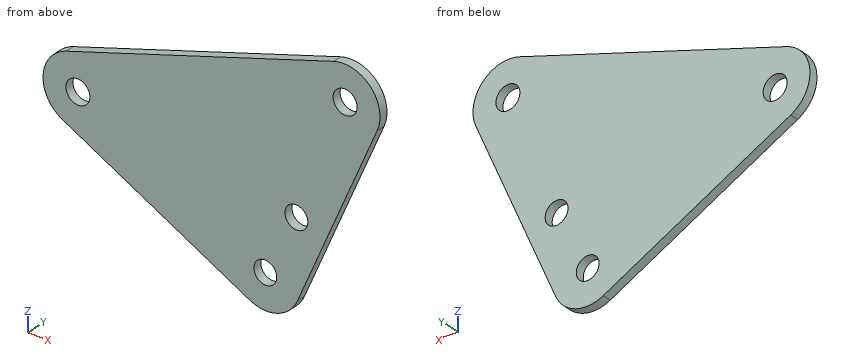
Autodesk Inventor part; units mm, degrees
ref_plane "YZ Plane" through (0, 0, 0) normal (1, 0, 0) x (0, 1, 0)
ref_plane "XZ Plane" through (0, 0, 0) normal (0, 1, 0) x (-1, 0, 0)
ref_plane "XY Plane" through (0, 0, 0) normal (0, 0, 1) x (1, 0, 0)
sketch "Sketch1" plane through (0, 0, 0) normal (0, 1, 0) x (-1, 0, 0)
  circle A0 centre (-25.0009, 13.9426) radius 2.1844
  circle A1 centre (-10.4764, -20.0504) radius 2.0828
  circle A2 centre (-16.132, -8.6792) radius 2.0828
  circle A3 centre (23.6373, -3.084) radius 2.1844
  arc A4 (-22.9029, 19.936) -> (-30.8402, 11.4476) centre (-25.0009, 13.9426) ccw
  arc A5 (-16.3157, -22.5454) -> (-7.6487, -25.736) centre (-10.4764, -20.0504) ccw
  arc A6 (26.4651, -8.7697) -> (25.7354, 2.9094) centre (23.6373, -3.084) ccw
  line L0 (-30.8402, 11.4476) -> (-16.3157, -22.5454)
  line L1 (-22.9029, 19.936) -> (25.7354, 2.9094)
  line L2 (26.4651, -8.7697) -> (-7.6487, -25.736)
  point P0 (0, 0)
extrude "Extrusion1" add sketch "Sketch1" along normal blind 1.5875
properties part number "newstackpoly"
Geometry check sheet. Reference: the model listing, model coordinates, mm. Give positions to 0.01 mm unless a question says otherwise; leave off trailing zeros. Write each loop counter-clockwise with the first axis right and the second up, starting at its lowest first coordinate (ties: lowest second). Pieces come first, ordered by that corner, then holes. Notation, with made-up numbers: (73.25, 81) - (113.25, 81) arc R14 cw to (113.25, 93) - close; hole circle Ø4 at (68.5, 86). An arc over 180 degrees is marked (long way). Put each result on its own line as item: value.
1. Sectioned sample at A-A, the plane z = -4. Enter the section's corners in (x, y), plus the area to 3 significant figures.
Ans:
outline: (-29.92, 0) - (-25.62, 0) - (-25.62, 1.59) - (-29.92, 1.59) - close; (-21.65, 0) - (24.24, 0) - (24.24, 1.59) - (-21.65, 1.59) - close
area: 79.7 mm²
2. Sectioned sample at C-C, the plane y = 0.7. Enter the section's corners in (x, z).
Ans:
outline: (-26.47, -8.77) - (7.65, -25.74) arc R6.35 ccw to (16.32, -22.55) - (30.84, 11.45) arc R6.35 ccw to (22.9, 19.94) - (-25.74, 2.91) arc R6.35 ccw to start; hole circle Ø4.37 at (-23.64, -3.08); hole circle Ø4.17 at (10.48, -20.05); hole circle Ø4.17 at (16.13, -8.68); hole circle Ø4.37 at (25, 13.94)
3. Sectioned sample at B-B, the plane x = -25. Enter the section's corners in (y, z), plus the area to 3 significant figures.
Ans:
outline: (0, -9.5) - (1.59, -9.5) - (1.59, -4.79) - (0, -4.79) - close; (0, -1.38) - (1.59, -1.38) - (1.59, 3.17) - (0, 3.17) - close
area: 14.7 mm²
4. Thickness scan on line 1 (X direction, y = 0.1, z = -20); line 2 (Z direction, x = 9.5, y = 1.5); line 3 (Z direction, x = 16, y = 0.95). Record the ranges inside material, lowest first.
Ans:
line 1: x = -3.88 to 8.39, 12.56 to 17.4
line 2: z = -26.32 to -21.89, -18.21 to 15.24
line 3: z = -23.18 to -10.76, -6.6 to 17.52
5. Sectioned sample at D-D, the plane x = -7.5. Enter the section's corners in (y, z).
Ans:
outline: (0, -18.2) - (1.59, -18.2) - (1.59, 9.29) - (0, 9.29) - close
